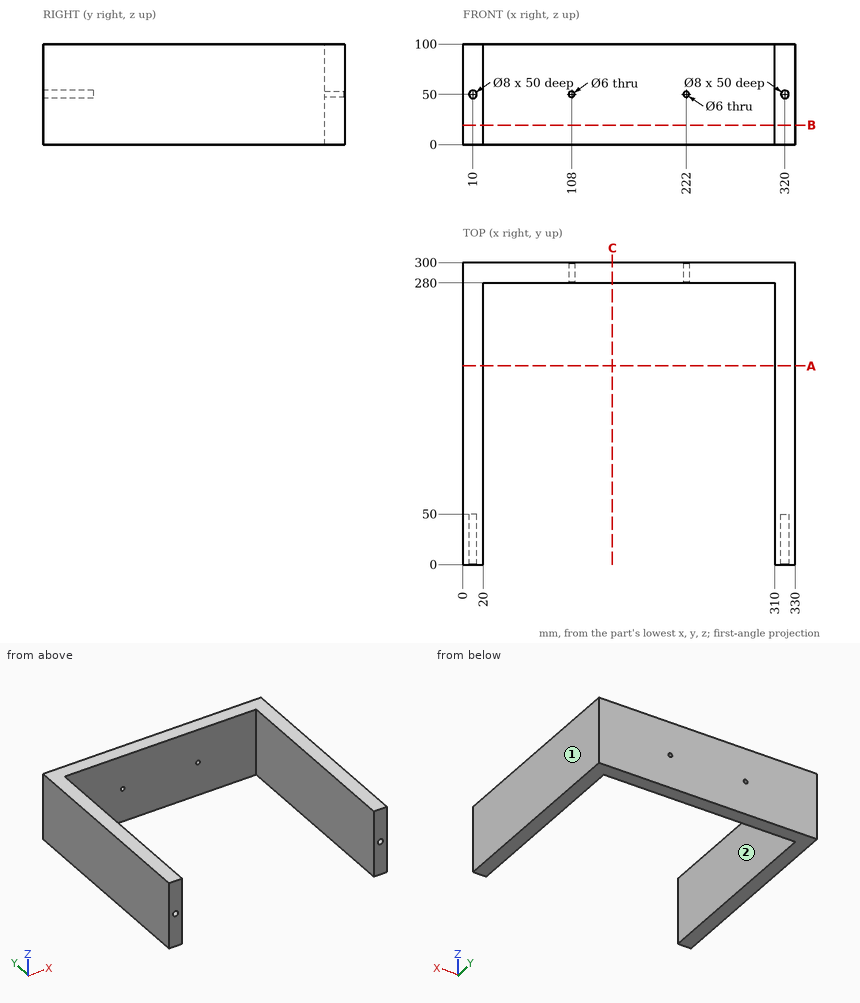
Geometry: see drawing. Coordinates: mm, zero at the bounding-box minimum. A direction names the side the tool comes from. Give positions to 0.01 mm unless a question says otherwise; leave off trailing zeros. Order: outer loops, then holes, each group sorted by start corner. A loop starts at its lowest first (then second) coordinate and runs counter-clockwise, first axis right, second up. Notation, with made-up numbers: (29.25, 21) - (35.25, 21) arc R31 cw to (35.25, 54) - close; hole circle Ø8 at (83.25, -18). An arc over 180 degrees is marked (long way). Write each question's results on one line, items separated by ' | '.
Item 1: Contact query for flat-ended pins moving along their axis: pin 1 Ø2.5 at (x, z) = (10.5, 52) entering from -Y; pin 2 Ø3 at (x, z) = (74, 36.5) entering from -Y. Output: stop coordinate, or through.
A:
pin 1: stops at y = 50 | pin 2: stops at y = 280
Item 2: Section C-C (x = 148.5). Return loops of the section in (y, z), and give its area (3 significant figures).
A:
outline: (280, 0) - (300, 0) - (300, 100) - (280, 100) - close | area: 2,000 mm^2
Item 3: Access query for the marked faces 1 and 2. Directions: +Z, -Z, +X, -X, +Y, -Y. A direction counts if a zero-diameter tool reaches every point of the face in a straight line with its end or side. Return the directions, or none.
A:
face 1: +Z, -Z, +X, +Y, -Y | face 2: +Z, -Z, -Y
Item 4: Section B-B (z = 19.5). Return loops of the section in (x, y), and give its area (3 significant figures).
A:
outline: (0, 0) - (20, 0) - (20, 280) - (310, 280) - (310, 0) - (330, 0) - (330, 300) - (0, 300) - close | area: 17,800 mm^2
Item 5: Material intervals for line 1 along X through (y, z) = (290, 50); line 2 along X through (y, z) = (131, 59); line 3 along Z through (x, y) = (320, 15), sorted ascending.
A:
line 1: x = 0 to 105, 111 to 219, 225 to 330 | line 2: x = 0 to 20, 310 to 330 | line 3: z = 0 to 46, 54 to 100
Item 6: Section A-A (y = 197.5). Return loops of the section in (x, z).
A:
outline: (0, 0) - (20, 0) - (20, 100) - (0, 100) - close; (310, 0) - (330, 0) - (330, 100) - (310, 100) - close
